Geometry: final body of the model. Coordinates: model frame, mm. Face numbers are marked on the shaded views. Give positions to 0.01 mm unless a question says otherwise; leave off trailing zeros. Loops run counter-clockwise (first coordinate to the right, second up) from the corner with the lowest first, then second, coordinate; pieces in that order, holes last.
1. Section C-C, the plane z = 1.55. Output: boundary loops of the cut face in (x, y), then the cut area to 3 significant figures.
2. Material intervals for line 1 along X through (y, z) = (-12.5, 2.2); line 2 along Y through (x, z) = (0, 0.5); line 3 along Y through (x, z) = (-11.5, 2.85), sorted ascending.
3. Section D-D, the plane y = 18. Output: boundary loops of the cut face in (x, z), then the cut area to 3 significant figures.
4. Draft query along X for the marked faces 1 and 2. Return one class per face: +X half, -X half, draft (parallel to the pull), parting line (faces both ways), or undercut.
5. First-contact query: P1, Ø1.5, axis at x = 20, z = 2, coming from the -Y side; P2, Ø0.9, axis at y = -11, z = 2, coming from the -X side; P3, Ø0.9, axis at x = 16, z = 1, coming from the +Y side. Flat tips, straight axial feed; report the tip coordinate or a pass-through.
6. Section A-A, the plane x = 0. Output: boundary loops of the cut face in (y, z).
7. Section B-B, the plane y = 0. Output: boundary loops of the cut face in (x, z), then the cut area to 3 significant figures.
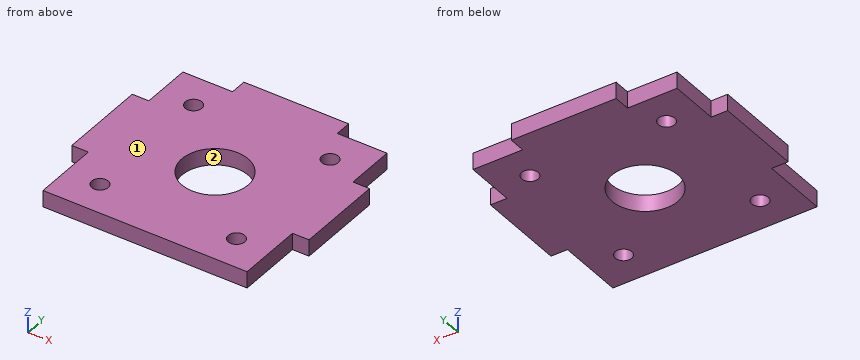
from build123d import *

# Parameters (mm, degrees)
SKETCH1_W           = 43
SKETCH1_H           = 43
SKETCH1_R           = 1.5
SKETCH1_R_2         = 6
BOSS_EXTRUDE1_DEPTH = 3
CUT_EXTRUDE1_DEPTH  = 3


with BuildPart() as part:
    # Sketch1 → Boss-Extrude1 (new body)
    with BuildSketch(Plane.XY):
        Rectangle(SKETCH1_W, SKETCH1_H)
        with Locations((-12.374368671, 12.374368671)):
            Circle(SKETCH1_R, mode=Mode.SUBTRACT)
        with Locations((12.374368671, -12.374368671)):
            Circle(SKETCH1_R, mode=Mode.SUBTRACT)
        with Locations((12.374368671, 12.374368671)):
            Circle(SKETCH1_R, mode=Mode.SUBTRACT)
        with Locations((-12.374368671, -12.374368671)):
            Circle(SKETCH1_R, mode=Mode.SUBTRACT)
        Circle(SKETCH1_R_2, mode=Mode.SUBTRACT)
    extrude(amount=BOSS_EXTRUDE1_DEPTH)

    # Sketch2 → Cut-Extrude1 (cut)
    with BuildSketch(Plane.XY.offset(3)):
        Polygon((-21.5, -21.5), (21.5, -21.5), (21.5, -18.5), (21.5, -6.5), (18.5, -6.5), (18.5, -18.5), (-18.5, -18.5), (-18.5, -6.5), (-21.5, -6.5), (-21.5, -18.5), align=None)
        Polygon((-21.5, 9.5), (-18.5, 9.5), (-18.5, 18.5), (-9.5, 18.5), (-9.5, 21.5), (-21.5, 21.5), align=None)
        Polygon((21.5, 9.5), (21.5, 21.5), (9.5, 21.5), (9.5, 18.5), (18.5, 18.5), (18.5, 9.5), align=None)
    extrude(amount=-CUT_EXTRUDE1_DEPTH, mode=Mode.SUBTRACT)


solid = part.part
Answers below:
1. outline: (-21.5, -6.5) - (-18.5, -6.5) - (-18.5, -18.5) - (18.5, -18.5) - (18.5, -6.5) - (21.5, -6.5) - (21.5, 9.5) - (18.5, 9.5) - (18.5, 18.5) - (9.5, 18.5) - (9.5, 21.5) - (-9.5, 21.5) - (-9.5, 18.5) - (-18.5, 18.5) - (-18.5, 9.5) - (-21.5, 9.5) - close; hole circle Ø3 at (-12.37, -12.37); hole circle Ø3 at (-12.37, 12.37); hole circle Ø12 at (0, 0); hole circle Ø3 at (12.37, -12.37); hole circle Ø3 at (12.37, 12.37)
1. area: 1,380 mm2
2. line 1: x = -18.5 to -13.87, -10.88 to 10.88, 13.87 to 18.5
2. line 2: y = -18.5 to -6, 6 to 21.5
2. line 3: y = -18.5 to -13.59, -11.16 to 11.16, 13.59 to 18.5
3. outline: (-18.5, 0) - (18.5, 0) - (18.5, 3) - (-18.5, 3) - close
3. area: 111 mm2
4. face 1: draft
4. face 2: undercut
5. P1: stops at y = -6.5
5. P2: stops at x = -18.5
5. P3: stops at y = 18.5
6. outline: (-18.5, 0) - (-6, 0) - (-6, 3) - (-18.5, 3) - close; (6, 0) - (21.5, 0) - (21.5, 3) - (6, 3) - close
7. outline: (-21.5, 0) - (-6, 0) - (-6, 3) - (-21.5, 3) - close; (6, 0) - (21.5, 0) - (21.5, 3) - (6, 3) - close
7. area: 93.0 mm2
